Could you check a few things on this model? Use its own coordinates, in mm. A direction names the side the tool comes from. Coordinates: 2 decimals unless noted, no trailing zeros. Order: outer loops, then holes, each group sorted by start corner. A loop starts at its lowest first (then second) coordinate and runs counter-clockwise, first axis right, second up. Notation, with made-up numbers: (-29, 53.25) - (-25, 53.25) arc R26 ccw to (-25, 91.25) - close; hole circle Ø7 at (86, 26). An arc over 180 degrees is marked (long way). One line per item, written item: value.
from build123d import *

# Parameters (mm, degrees)
F0_W     = 300
F0_H     = 50
F1_DEPTH = 15
F2_W     = 50
F2_H     = 10
F3_DEPTH = 15.001
F5_W     = 40
F5_H     = 15
F6_DEPTH = 5
F7_W     = 70
F7_H     = 10
F8_DEPTH = 5


with BuildPart() as f1:
    # F0 (on Top) → F1 (new body)
    with BuildSketch(Plane.XY):
        Rectangle(F0_W, F0_H)
    extrude(amount=F1_DEPTH)

    # F2 (on face) → F3 (cut, through all)
    with BuildSketch(Plane.XY.offset(15)):
        with Locations((0, 20)):
            Rectangle(F2_W, F2_H)
    extrude(amount=-F3_DEPTH, mode=Mode.SUBTRACT)

    # F5 (on face) → F6 (join)
    with BuildSketch(Plane(origin=(0, 25, 0), x_dir=(-1, 0, 0), z_dir=(0, 1, 0))):
        with Locations((30, 7.5)):
            Rectangle(F5_W, F5_H)
    extrude(amount=F6_DEPTH)

    # F7 (on face) → F8 (cut)
    with BuildSketch(Plane.XY.offset(15)):
        with Locations((-95, 15)):
            Rectangle(F7_W, F7_H)
    extrude(amount=-F8_DEPTH, mode=Mode.SUBTRACT)


solid = f1.part
Item 1: I want a section at B-B on z = 6.25. Please give me the cut outline in (x, y).
Conclusion:
outline: (-150, -25) - (150, -25) - (150, 25) - (25, 25) - (25, 15) - (-25, 15) - (-25, 25) - (-10, 25) - (-10, 30) - (-50, 30) - (-50, 25) - (-150, 25) - close
Item 2: I'm going to push flat-ended pins straight in: pin 1 Ø4 at (x, y) = (63, -3) entering from -Z; pin 2 Ø8 at (x, z) = (71.5, 7) entering from +Y; pin 3 Ø4 at (y, z) = (28, 4) entering from +X; pin 4 Ø5 at (x, y) = (-87, 15) entering from +Z. Where does each tip first touch, or does it pass through?
Conclusion:
pin 1: z = 0
pin 2: y = 25
pin 3: x = -10
pin 4: z = 10
Item 3: I want a section at C-C on x = 17. Please give me the cut outline in (y, z), then the cut area to 3 significant figures.
Conclusion:
outline: (-25, 0) - (15, 0) - (15, 15) - (-25, 15) - close
area: 600 mm²
Item 4: I want a section at A-A on x = -104.5. Please give me the cut outline in (y, z).
Conclusion:
outline: (-25, 0) - (25, 0) - (25, 15) - (20, 15) - (20, 10) - (10, 10) - (10, 15) - (-25, 15) - close
Item 5: For faces 1 (the face through (-17, 25, 8)), 2 (the face through (-95, 10, 13)), 3 (the face through (25, 20, 8)), which set-ups out of +Z, -Z, +X, -X, +Y, -Y let a thin tool reach every point of the face, with its end or its side?
Conclusion:
face 1: +Z, -Z
face 2: +Z
face 3: +Z, -Z, +Y
Item 6: If I drill on probe 1 along X at (y, z) = (24.5, 9); probe 2 along Y at (x, z) = (-127, 0.75); probe 3 along Y at (x, z) = (-11.5, 12.5), over which ranges is the centre line in solid material (lowest first)?
Conclusion:
probe 1: -150 to -25, 25 to 150
probe 2: -25 to 25
probe 3: -25 to 15, 25 to 30
Item 7: Thinking about a two-plate mould opening in X: for faces 4 (the face through (2, 2, 0)), 5 (the face through (-95, 20, 13)), 6 (the face through (150, 0, 7)), which applies, pulls with the +X half, pulls with the -X half, needs draft (parallel to the pull), parting line crosses it, or undercut?
Conclusion:
face 4: needs draft
face 5: undercut
face 6: pulls with the +X half
